CAD build for the part. Positions are in the model's coordinates, mm. A direction names the side the tool comes from. Round coordinates to 2 decimals unless told otherwise and drop trailing zeros. Loops run counter-clockwise (first coordinate to the right, second up) from the corner with the lowest first, then second, coordinate; pieces in that order, holes last.
from build123d import *

# Parameters (mm, degrees)
SKETCH_1_W           = 20
SKETCH_1_H           = 20
BASEBOX_DEPTH        = 10
SKETCH_2_W           = 5
SKETCH_2_H           = 5
TARGETBOX_DEPTH      = 10
SKETCH_3_R           = 3
UPTOVERTEXBOSS_DEPTH = 20


with BuildPart() as part:
    # 草图1 → BaseBox (new body)
    with BuildSketch(Plane.XY):
        with Locations((10, 10)):
            Rectangle(SKETCH_1_W, SKETCH_1_H)
    extrude(amount=BASEBOX_DEPTH)



with BuildPart() as body_2:
    # 草图2 → TargetBox (new body)
    with BuildSketch(Plane.XY.offset(20)):
        with Locations((5.5, 5.5)):
            Rectangle(SKETCH_2_W, SKETCH_2_H)
    extrude(amount=TARGETBOX_DEPTH)


with BuildPart() as part_1:
    add(part.part)

    add(body_2.part)  # UpToVertexBoss merges body 2
    # 草图3 → UpToVertexBoss (add)
    with BuildSketch(Plane.XY.offset(10)):
        with Locations(Location((10, 10, 0), (0, 0, 221.810314896))):
            Circle(SKETCH_3_R)
    extrude(amount=UPTOVERTEXBOSS_DEPTH)


solid = part_1.part
Item 1: 3-axis set-ups, long thin cutter, end or side, ignore diameter. For faces 1 (the flat face through (3, 5, 25)), 2 (the flat face through (5, 3, 25)), 3 (the flat face through (7.6, 12.4, 10)): which of +Z, -Z, +X, -X, +Y, -Y reach the whole face in a straight line?
Verdict:
face 1: +Z, -X, +Y, -Y
face 2: +Z, +X, -X, -Y
face 3: none
Item 2: Flat gauge pins, fed straight in: P1, Ø8, axis at x = 3, y = 14, coming from the +Z side; P2, Ø2.5, axis at y = 5, z = 23, coming from the -X side; P3, Ø5.5, axis at x = 4.5, z = 24, coming from the -Y side. Where does each tip first touch, or does it go through?
Verdict:
P1: stops at z = 10
P2: stops at x = 3
P3: stops at y = 3
Item 3: Cut at B-B (z = 21.25). List the corners of the cut face in (x, y), plus the area to 3 significant figures.
Verdict:
outline: (3, 3) - (8, 3) - (8, 7.76) arc R3 ccw (long way) to (7.76, 8) - (3, 8) - close
area: 53.2 mm2
Item 4: Cut at A-A (x = 5.5). List the corners of the cut face in (y, z).
Verdict:
outline: (0, 0) - (20, 0) - (20, 10) - (0, 10) - close; (3, 20) - (8, 20) - (8, 30) - (3, 30) - close
Item 5: Wall check: L1, parallel to Z at x = 7.75, y = 14.5; L2, parallel to X at y = 10, z = 23.75; L3, parallel to X at y = 8.5, z = 23.5. Give the ranges that are in metal, low to high.
Verdict:
L1: z = 0 to 10
L2: x = 7 to 13
L3: x = 7.4 to 12.6
Item 6: Mould opens along Z. For faces 4 (the flat face through (0, 10, 5)), 5 (the flat face through (5, 6, 20)), 6 (the flat face through (7.8, 7.5, 30)), 7 (the flat face through (10, 10, 0)) say: released by +Z, released by -Z, zero draft, split by the parting line, or undercut.
Verdict:
face 4: zero draft
face 5: undercut
face 6: released by +Z
face 7: released by -Z
Item 7: Cut at C-C (y = 10). List the corners of the cut face in (x, z).
Verdict:
outline: (0, 0) - (20, 0) - (20, 10) - (13, 10) - (13, 30) - (7, 30) - (7, 10) - (0, 10) - close
